Read the model definition and answer for the solid it produces. Units are mm, in the model's axes. A direction names the side the tool comes from. Round coordinates to 2 decimals unless told otherwise and drop trailing zeros. Loops run counter-clockwise (first coordinate to the right, second up) from the corner with the lowest first, then second, coordinate; pieces in that order, holes last. Notation, with made-up numbers: (65, 67.5) - (117, 67.5) arc R20 cw to (117, 98.5) - close; hole circle Ø5 at (42.25, 28). An arc over 180 degrees is marked (long way). Use CSV: the item, a comma, the result in double quotes. Start each with the question number.
1. Find section D-D (z = 40). Give the vertices of the cut face in (x, y), and give its area (3 significant figures).
2. Find section C-C (y = 15). Give the vertices of the cut face in (x, z).
3. Given pin 1 Ø13.5 at (y, z) = (-15.5, 35.5) entering from +X; pin 2 Ø1 at (y, z) = (1.5, 82.5) entering from +X; pin 3 Ø8 at (x, z) = (36.5, 2) entering from +Y, each flat-ended and moving along its own axis, determine where each tip first touches the part or whether it passes through.
4. A tool of negligible diameter and unlimited length cuts with its end or side. For faces 5 (the cylindrical face through (32.72, -0.41, 117.6)), 6 (the flat face through (4.242, -9.689, -29.881)), from which of +Z, -Z, +X, -X, +Y, -Y can it reach the whole face along a straight path? Write none if from no direction.
5. Consider line 1 along Z through (x, y) = (-27.5, -17); line 2 along X through (y, z) = (-18, -26); line 3 along Y through (x, z) = (-26.5, 14). Determine where each line is inside the solid, lowest interval first.
6. Find section A-A (y = -18). Give the vertices of the cut face in (x, z).
7. Determine the mould class of faces 1 (the flat face through (-48, 29, -94)), 2 (the flat face through (31.13, -9.69, 5.3)), 3 (the cylindrical face through (-180.813, 2.636, 3.313)), 4 (the cylindrical face through (-186.459, -0.406, 5.586)) for opening direction Z: +Z half, -Z half, draft (parallel to the pull), parting line (faces both ways), or undercut.
8. Find section B-B (x = 19). Give the vertices of the cut face in (y, z).
from build123d import *

# Parameters (mm, degrees)
F1_DEPTH = 29
F2_T     = -6
F3_DEPTH = 25


with BuildPart() as f1:
    # F0 (on Front) → F1 (new body, symmetric)
    with BuildSketch(Plane.XZ):
        with BuildLine():
            ThreePointArc((-120.8260423411, 51.4157625441), (-187.0617060927, 4.5833458701), (-196.3255107403, -76.005861395))
            Line((-196.3255107403, -76.005861395), (-196.3255107403, -98.1331872754))
            Line((-196.3255107403, -98.1331872754), (131.9251656532, -98.1331872754))
            Line((131.9251656532, -98.1331872754), (131.9251656532, -12.0712618296))
            ThreePointArc((131.9251656532, -12.0712618296), (30.305701886, 118.2300959975), (-120.8260423411, 51.4157625441))
        make_face()
        Polygon((-6.9567829963, 7.8355963742), (7.4647014605, 29.7945929541), (7.4647014605, 5.8520050569), (29.8372825252, -0.5733477102), (5.157555885, -9.4960665254), (-1.5632266534, -28.2956225947), (-9.7149439706, -5.7484417182), (-30.2154383046, -0.5733477102), align=None, mode=Mode.SUBTRACT)
    extrude(amount=F1_DEPTH, both=True)

    # F2
    f2_openings = [f1.faces().sort_by_distance(p)[0] for p in [
        (-24.069306, 29, -4.408664),
    ]]
    offset(amount=F2_T, openings=f2_openings, kind=Kind.INTERSECTION)

    # F3 (cut): a face of the model
    f3_faces = [f1.faces().sort_by_distance(p)[0] for p in [
        (2.4525988659, 29, 30.5693044377),
    ]]
    extrude(f3_faces, amount=-F3_DEPTH, mode=Mode.SUBTRACT)


solid = f1.part
Filled sheet:
1,outline,"(-151.23, -29) - (121.42, -29) - (121.42, 29) - (114.89, 29) - (114.89, -23) - (13.46, -23) - (13.46, 4) - (6.99, 4) - (6.99, -23) - (-137.76, -23) - (-137.76, 29) - (-151.23, 29) - close"
1,area,"2,850 mm²"
2,outline,"(-196.33, -98.13) - (131.93, -98.13) - (131.93, -12.07) arc R134.35 ccw to (-120.83, 51.42) arc R99.37 ccw to (-196.33, -76.01) - close; hole (-190.33, -92.13) - (125.93, -92.13) - (125.93, -12.07) arc R128.35 ccw to (-116.87, 46.04) arc R93.37 ccw to (-190.33, -75.07) - close"
3,pin 1,"stops at x = 125.57"
3,pin 2,"stops at x = 93.49"
3,pin 3,"stops at y = 4"
4,face 5,"+Z, +Y, -Y"
4,face 6,"+Y"
5,line 1,"z = -98.13 to -92.13, -7.45 to -1.26, 0.41 to 6.79, 113.8 to 119.92"
5,line 2,"x = -198.89 to -192.76, -8.77 to -2.39, -0.74 to 5.63, 125.93 to 131.93"
5,line 3,"y = -29 to -23"
6,outline,"(-196.33, -98.13) - (131.93, -98.13) - (131.93, -12.07) arc R134.35 ccw to (-120.83, 51.42) arc R99.37 ccw to (-196.33, -76.01) - close; (-50.69, -1.59) - (-14.27, -10.79) - (-1.53, -46.03) - (9.86, -14.18) - (49.29, 0.08) - (13.46, 10.37) - (13.46, 49.86) - (-10.88, 12.8) - close; hole (-190.33, -92.13) - (125.93, -92.13) - (125.93, -12.07) arc R128.35 ccw to (-116.87, 46.04) arc R93.37 ccw to (-190.33, -75.07) - close; hole (-30.22, -0.57) - (-9.71, -5.75) - (-1.56, -28.3) - (5.16, -9.5) - (29.84, -0.57) - (7.46, 5.85) - (7.46, 29.79) - (-6.96, 7.84) - close"
7,face 1,"draft"
7,face 2,"undercut"
7,face 3,"undercut"
7,face 4,"parting line"
8,outline,"(-29, -98.13) - (29, -98.13) - (29, -92.13) - (-23, -92.13) - (-23, -10.87) - (4, -10.87) - (4, -4.49) - (-29, -4.49) - close; (-29, 2.54) - (4, 2.54) - (4, 8.78) - (-23, 8.78) - (-23, 114.48) - (29, 114.48) - (29, 120.56) - (-29, 120.56) - close"
